CAD build for the part. Positions are in the model's coordinates, mm. Face numbers are marked on the shaded views. A direction names the side the tool comes from. Give positions to 0.01 mm unless a question says otherwise; leave off trailing zeros. Write each loop counter-clockwise with the first axis right and the second up, starting at its lowest first coordinate (ties: lowest second). Pieces come first, ordered by that corner, then holes. Notation, with made-up numbers: (-22.75, 89) -> (-8.75, 89) arc R25 ccw to (-8.75, 102) -> close; hole circle Ø9 at (-38.75, 66). An arc over 180 degrees is marked (long way). Answer as a JSON object with one key per item and string values.
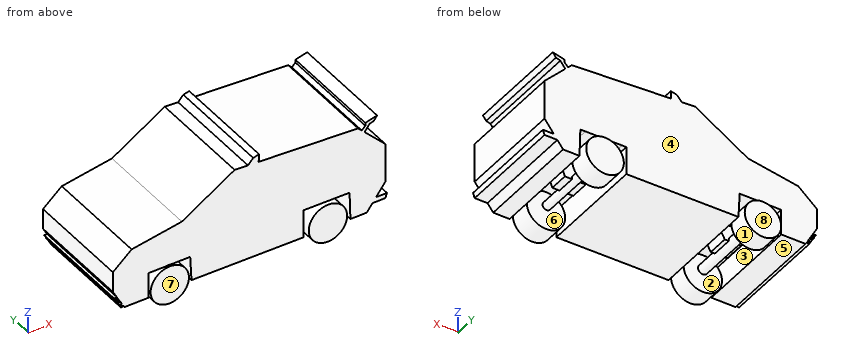
```python
from build123d import *

# Parameters (mm, degrees)
F1_DEPTH       = 25.4
F4_DEPTH       = 2.54
F4_DEPTH_BACK  = 2.54
F7_DEPTH       = 2.032
F7_DEPTH_BACK  = 2.54
F8_R           = 1.1576826641
F9_DEPTH       = 12.7
F9_DEPTH_BACK  = 12.7
F10_R          = 0.9804880259
F11_DEPTH      = 12.7
F11_DEPTH_BACK = 12.7
F13_R          = 4.572
F14_DEPTH      = 4.572
F15_R          = 4.572
F16_DEPTH      = 5.08
F18_R          = 4.4779357242
F19_DEPTH      = 5.08
F20_R          = 4.3509487434
F21_DEPTH      = 4.826
F22_DEPTH      = 25.4
F23_DEPTH      = 25.4


with BuildPart() as f1:
    # F0 (on Front) → F1 (new body)
    with BuildSketch(Plane.XZ):
        Polygon((-42.7369444011, 4.6772318892), (-36.9589328766, 4.6772318892), (-36.9589328766, 10.7693634927), (-27.0514115691, 10.7693634927), (-26.7468057573, 4.8803025857), (0, 4.6772318892), (0, 11.3719804212), (1.0606472588, 11.3639276325), (9.7543726708, 11.297921961), (10.9652050924, 11.2887289162), (11.1689083278, 4.6772318892), (15.0829743681, 4.6772318892), (16.4426990051, 6.4901970327), (17.2888992398, 7.6184633654), (19.4948241115, 10.5596948415), (19.4948241115, 19.900964573), (14.554232661, 24.8415538992), (13.8758348479, 25.5199514207), (12.9965478554, 26.3992380351), (-10.717479028, 27.7076002598), (-13.2646739035, 27.8481353773), (-16.4487566799, 28.0238091946), (-29.0391631424, 20.3071068972), (-41.0203561187, 18.2763971388), (-45.4879179597, 14.4180459902), (-45.4879179597, 9.5443399623), (-44.5200988283, 7.8320442214), (-44.3530531096, 7.5365017348), (-44.1124311804, 7.1107859258), (-43.9645371878, 6.8491272694), (-43.8518225557, 6.6497090328), (-43.6986885549, 6.3787795906), (-43.3529015226, 5.7670024068), (-43.17437928, 5.4511552968), (-42.9887916429, 5.122807871), align=None)
        Polygon((-43.5131009178, 4.8264592117), (-42.9887916429, 5.122807871), (-43.17437928, 5.4511552968), (-43.6986885549, 5.1548066375), align=None)
        Polygon((-43.8739407822, 5.4511552968), (-43.17437928, 5.4511552968), (-43.3529015226, 5.7670024068), (-44.0524630249, 5.7670024068), align=None)
        Polygon((-44.4116123194, 6.3787795906), (-43.6986885549, 6.3787795906), (-43.8518225557, 6.6497090328), (-44.5647463202, 6.6497090328), align=None)
        Polygon((-44.7156839396, 6.8491272694), (-43.9645371878, 6.8491272694), (-44.1124311804, 7.1107859258), (-44.8635779321, 7.1107859258), align=None)
        Polygon((-45.0380556521, 7.5365017348), (-44.3530531096, 7.5365017348), (-44.5200988283, 7.8320442214), (-45.2051013708, 7.8320442214), align=None)
        Polygon((17.2888992398, 7.6184633654), (16.4426990051, 6.4901970327), (19.4948241115, 6.4901970327), (19.8960918933, 7.6184633654), align=None)
        Polygon((13.8758348479, 25.5199514207), (14.554232661, 24.8415538992), (15.7266985625, 26.4048408717), (16.7735743968, 26.7441401112), (17.537901178, 27.763241902), (14.7154445676, 27.0689483732), (14.7154445676, 26.3595615014), align=None)
        Polygon((-12.0249697939, 29.2020086199), (-13.2646739035, 27.8481353773), (-10.717479028, 27.7076002598), (-10.6161860749, 29.5435320586), align=None)
    extrude(amount=F1_DEPTH)

    # F3 (on offset) → F4 (join, two sides)
    with BuildSketch(Plane.XZ.offset(12.7)) as f4_sk:
        Polygon((-28.008485968, 10.7693634927), (-35.8356192608, 10.7693634927), (-34.0407073398, 6.9641508162), (-30.1636971433, 6.9641508162), align=None)
    extrude(amount=F4_DEPTH)
    extrude(f4_sk.sketch, amount=-F4_DEPTH_BACK)

    # F6 (on offset) → F7 (join, two sides)
    with BuildSketch(Plane.XZ.offset(12.7)) as f7_sk:
        Polygon((9.4945231002, 11.2998948258), (0.8765038544, 11.3653257108), (2.9983955901, 7.1409773082), (7.989410311, 7.1365474723), align=None)
    extrude(amount=F7_DEPTH)
    extrude(f7_sk.sketch, amount=-F7_DEPTH_BACK)

    # F8 (on offset) → F9 (join, two sides)
    with BuildSketch(Plane.XZ.offset(12.7)) as f9_sk:
        with Locations((-32.2571918368, 7.1993744932)):
            Circle(F8_R)
    extrude(amount=F9_DEPTH)
    extrude(f9_sk.sketch, amount=-F9_DEPTH_BACK)

    # F10 (on offset) → F11 (join, two sides)
    with BuildSketch(Plane.XZ.offset(12.7)) as f11_sk:
        with Locations((5.3251022473, 7.4197696522)):
            Circle(F10_R)
    extrude(amount=F11_DEPTH)
    extrude(f11_sk.sketch, amount=-F11_DEPTH_BACK)

    # F13 (on offset) → F14 (join)
    with BuildSketch(Plane.XZ.offset(25.908)):
        with Locations((-32.2608351707, 6.2622600235)):
            Circle(F13_R)
    extrude(amount=-F14_DEPTH)

    # F15 (on offset) → F16 (join)
    with BuildSketch(Plane.XZ.offset(25.908)):
        with Locations((5.4841622319, 6.2622600235)):
            Circle(F15_R)
    extrude(amount=-F16_DEPTH)

    # F18 (on offset) → F19 (join)
    with BuildSketch(Plane.XZ.offset(-0.5842)):
        with Locations((5.4573472589, 6.6700675525)):
            Circle(F18_R)
    extrude(amount=F19_DEPTH)

    # F20 (on offset) → F21 (join)
    with BuildSketch(Plane.XZ.offset(-0.5842)):
        with Locations((-32.2135724127, 6.1565306969)):
            Circle(F20_R)
    extrude(amount=F21_DEPTH)

    # F0 (on Front) → F22 (join)
    with BuildSketch(Plane.XZ):
        Polygon((-42.7369444011, 4.6772318892), (-36.9589328766, 4.6772318892), (-36.9589328766, 10.7693634927), (-27.0514115691, 10.7693634927), (-26.7468057573, 4.8803025857), (0, 4.6772318892), (0, 11.3719804212), (1.0606472588, 11.3639276325), (9.7543726708, 11.297921961), (10.9652050924, 11.2887289162), (11.1689083278, 4.6772318892), (15.0829743681, 4.6772318892), (16.4426990051, 6.4901970327), (17.2888992398, 7.6184633654), (19.4948241115, 10.5596948415), (19.4948241115, 19.900964573), (14.554232661, 24.8415538992), (13.8758348479, 25.5199514207), (12.9965478554, 26.3992380351), (-10.717479028, 27.7076002598), (-13.2646739035, 27.8481353773), (-16.4487566799, 28.0238091946), (-29.0391631424, 20.3071068972), (-41.0203561187, 18.2763971388), (-45.4879179597, 14.4180459902), (-45.4879179597, 9.5443399623), (-44.5200988283, 7.8320442214), (-44.3530531096, 7.5365017348), (-44.1124311804, 7.1107859258), (-43.9645371878, 6.8491272694), (-43.8518225557, 6.6497090328), (-43.6986885549, 6.3787795906), (-43.3529015226, 5.7670024068), (-43.17437928, 5.4511552968), (-42.9887916429, 5.122807871), align=None)
        Polygon((-43.5131009178, 4.8264592117), (-42.9887916429, 5.122807871), (-43.17437928, 5.4511552968), (-43.6986885549, 5.1548066375), align=None)
        Polygon((-43.8739407822, 5.4511552968), (-43.17437928, 5.4511552968), (-43.3529015226, 5.7670024068), (-44.0524630249, 5.7670024068), align=None)
        Polygon((-44.4116123194, 6.3787795906), (-43.6986885549, 6.3787795906), (-43.8518225557, 6.6497090328), (-44.5647463202, 6.6497090328), align=None)
        Polygon((-44.7156839396, 6.8491272694), (-43.9645371878, 6.8491272694), (-44.1124311804, 7.1107859258), (-44.8635779321, 7.1107859258), align=None)
        Polygon((-45.0380556521, 7.5365017348), (-44.3530531096, 7.5365017348), (-44.5200988283, 7.8320442214), (-45.2051013708, 7.8320442214), align=None)
        Polygon((17.2888992398, 7.6184633654), (16.4426990051, 6.4901970327), (19.4948241115, 6.4901970327), (19.8960918933, 7.6184633654), align=None)
        Polygon((13.8758348479, 25.5199514207), (14.554232661, 24.8415538992), (15.7266985625, 26.4048408717), (16.7735743968, 26.7441401112), (17.537901178, 27.763241902), (14.7154445676, 27.0689483732), (14.7154445676, 26.3595615014), align=None)
        Polygon((-12.0249697939, 29.2020086199), (-13.2646739035, 27.8481353773), (-10.717479028, 27.7076002598), (-10.6161860749, 29.5435320586), align=None)
    extrude(amount=F22_DEPTH)

    # F0 (on Front) → F23 (join)
    with BuildSketch(Plane.XZ):
        Polygon((-42.7369444011, 4.6772318892), (-36.9589328766, 4.6772318892), (-36.9589328766, 10.7693634927), (-27.0514115691, 10.7693634927), (-26.7468057573, 4.8803025857), (0, 4.6772318892), (0, 11.3719804212), (1.0606472588, 11.3639276325), (9.7543726708, 11.297921961), (10.9652050924, 11.2887289162), (11.1689083278, 4.6772318892), (15.0829743681, 4.6772318892), (16.4426990051, 6.4901970327), (17.2888992398, 7.6184633654), (19.4948241115, 10.5596948415), (19.4948241115, 19.900964573), (14.554232661, 24.8415538992), (13.8758348479, 25.5199514207), (12.9965478554, 26.3992380351), (-10.717479028, 27.7076002598), (-13.2646739035, 27.8481353773), (-16.4487566799, 28.0238091946), (-29.0391631424, 20.3071068972), (-41.0203561187, 18.2763971388), (-45.4879179597, 14.4180459902), (-45.4879179597, 9.5443399623), (-44.5200988283, 7.8320442214), (-44.3530531096, 7.5365017348), (-44.1124311804, 7.1107859258), (-43.9645371878, 6.8491272694), (-43.8518225557, 6.6497090328), (-43.6986885549, 6.3787795906), (-43.3529015226, 5.7670024068), (-43.17437928, 5.4511552968), (-42.9887916429, 5.122807871), align=None)
        Polygon((-43.5131009178, 4.8264592117), (-42.9887916429, 5.122807871), (-43.17437928, 5.4511552968), (-43.6986885549, 5.1548066375), align=None)
        Polygon((-43.8739407822, 5.4511552968), (-43.17437928, 5.4511552968), (-43.3529015226, 5.7670024068), (-44.0524630249, 5.7670024068), align=None)
        Polygon((-44.4116123194, 6.3787795906), (-43.6986885549, 6.3787795906), (-43.8518225557, 6.6497090328), (-44.5647463202, 6.6497090328), align=None)
        Polygon((-44.7156839396, 6.8491272694), (-43.9645371878, 6.8491272694), (-44.1124311804, 7.1107859258), (-44.8635779321, 7.1107859258), align=None)
        Polygon((-45.0380556521, 7.5365017348), (-44.3530531096, 7.5365017348), (-44.5200988283, 7.8320442214), (-45.2051013708, 7.8320442214), align=None)
        Polygon((17.2888992398, 7.6184633654), (16.4426990051, 6.4901970327), (19.4948241115, 6.4901970327), (19.8960918933, 7.6184633654), align=None)
        Polygon((13.8758348479, 25.5199514207), (14.554232661, 24.8415538992), (15.7266985625, 26.4048408717), (16.7735743968, 26.7441401112), (17.537901178, 27.763241902), (14.7154445676, 27.0689483732), (14.7154445676, 26.3595615014), align=None)
        Polygon((-12.0249697939, 29.2020086199), (-13.2646739035, 27.8481353773), (-10.717479028, 27.7076002598), (-10.6161860749, 29.5435320586), align=None)
    extrude(amount=F23_DEPTH)


solid = f1.part
```
1) Pin check, flat tips, straight feed: pin 1 (12 mm diameter, centred on x = -34, z = 17, fed in from -Y); pin 2 (0.6 mm diameter, centred on x = -44, y = -17, fed in from +Z); pin 3 (5 mm diameter, centred on x = -20, z = 24.5, fed in from +Y). Stop position of each tip, or through.
Model answer:
{"pin 1": "stops at y = -25.4", "pin 2": "stops at z = 15.96", "pin 3": "stops at y = 0"}
2) Slice it at C-C (x = -25). List the corners of the cut face in (y, z).
Model answer:
{"outline": "(-25.4, 4.87) -> (0, 4.87) -> (0, 22.78) -> (-25.4, 22.78) -> close"}
3) Slice it at B-B (y = -16.75). State how many separate pieces and enclosed holes the cut face has, then the cut area to 3 significant figures.
Model answer:
{"separate pieces": "3", "enclosed holes": "0", "area": "1,120 mm2"}
4) Wall check: probe 1 along X at (y, z) = (-19.25, 5.25); probe 2 along Y at (x, z) = (-8.5, 13); probe 3 along X at (y, z) = (-24, 10.25). Give the ranges that are in metal, low to high.
Model answer:
{"probe 1": "x = -43.53 to -36.96, -26.77 to 0, 11.15 to 15.51", "probe 2": "y = -25.4 to 0", "probe 3": "x = -45.49 to -36.96, -34.5 to -30.02, -27.02 to 0, 3.25 to 7.72, 11 to 19.26"}
5) Mould opens along Y. For the marked faces 6, 7 and 8 say: released by +Y, released by -Y, zero draft, split by the parting line, or undercut.
Model answer:
{"face 6": "undercut", "face 7": "released by -Y", "face 8": "released by +Y"}
6) Slice it at A-A (z = 13.5). List the corners of the cut face in (x, y).
Model answer:
{"outline": "(-45.49, -25.4) -> (19.49, -25.4) -> (19.49, 0) -> (-45.49, 0) -> close"}
7) 3-axis set-ups, long thin cutter, end or side, ignore diameter. For the marked faces 1, 2, 3, 4 and 5: which of +Z, -Z, +X, -X, +Y, -Y reach the whole face in a straight line?
Model answer:
{"face 1": "+Y", "face 2": "none", "face 3": "-Z, +Y, -Y", "face 4": "+Z, +Y", "face 5": "-Z, -X, +Y, -Y"}
